Can you work these out from the model? Positions are in its coordinate system, mm. A direction names the side the tool comes from. Give positions to 0.01 mm unless a question says otherwise; leave off trailing zeros. Loops run counter-clockwise (first coordinate to the right, second up) from the corner with the lowest first, then second, coordinate; pieces in that order, holes last. Notation, with made-up numbers: (-14, -32) -> (18, -32) arc R20 ccw to (18, -27) -> close; hole circle Ø8 at (-1.5, 19). An arc over 180 degrees is marked (long way). Use CSV: the item, a comma, the result in double quotes.
from build123d import *

# Parameters (mm, degrees)
F0_W        = 45
F0_H        = 70
F1_DEPTH    = 3
F2_W        = 45
F2_H        = 4
F3_DEPTH    = 30
F4_T1_DEPTH = 119
F5_W        = 45
F5_H        = 3
F6_DEPTH    = 20
F7_R        = 5


# Not quite as in the source:
# - a fillet or chamfer that OpenCascade refuses, or shapes differently, is made with other operations: its cross-section is extruded or revolved along the edge and cut away or added


with BuildPart() as f1:
    # F0 (on Top) → F1 (new body)
    with BuildSketch(Plane.XY):
        Rectangle(F0_W, F0_H)
    extrude(amount=F1_DEPTH)

    # F2 (on face) → F3 (join)
    with BuildSketch(Plane.XY.offset(3)):
        with Locations((0, 33)):
            Rectangle(F2_W, F2_H)
    extrude(amount=F3_DEPTH)

    # F4: fillet of radius 23 on 2 edges, made by hand

    # F4_s2 → F4_t1 (cut)
    with BuildSketch(Plane.XZ.offset(-92.5)):
        with BuildLine():
            ThreePointArc((-22.5, 10), (-15.7634559673, 26.2634559673), (0.5, 33))
            Line((0.5, 33), (-22.5, 33))
            Line((-22.5, 33), (-22.5, 10))
        make_face()
        with BuildLine():
            ThreePointArc((-0.5, 33), (15.7634559673, 26.2634559673), (22.5, 10))
            Line((22.5, 10), (22.5, 33))
            Line((22.5, 33), (-0.5, 33))
        make_face()
    extrude(amount=F4_T1_DEPTH, mode=Mode.SUBTRACT)

    # F5 (on face) → F6 (join)
    with BuildSketch(Plane.XY.offset(3)):
        with Locations((0, -33.5)):
            Rectangle(F5_W, F5_H)
    extrude(amount=F6_DEPTH)

    # F7
    f7_edges = [f1.edges().sort_by_distance(p)[0] for p in [
        (-22.5, -33.5, 23),
        (22.5, -33.5, 23),
    ]]
    fillet(f7_edges, radius=F7_R)


solid = f1.part
(1) If we section it at D-D, the plane z = 14: Write out the boundary of the cut face in (x, y), then the cut area to 3 significant figures.
Answer sheet:
outline,"(-22.5, -35) -> (22.5, -35) -> (22.5, -32) -> (-22.5, -32) -> close; (-22.15, 31) -> (22.15, 31) -> (22.15, 35) -> (-22.15, 35) -> close"
area,"312 mm2"
(2) Will these pins go through, and if not, where does the flat tip stop? pin 1 Ø2 at (y, z) = (-4, 5) entering from -X; pin 2 Ø8 at (x, y) = (8.5, 11) entering from +Z; pin 3 Ø1.5 at (x, y) = (-8, -33.5) entering from +Z.
Answer sheet:
pin 1,"passes through"
pin 2,"stops at z = 3"
pin 3,"stops at z = 23"
(3) Which directions (+Z, -Z, +X, -X, +Y, -Y) give clear straight access to the entire face, cutting with the end or side of a thin tool? Please do faces 5 (the face through (0, -33, 23)), 6 (the face through (0, 0, 0)), 7 (the face through (0, 31, 14)), 8 (the face through (-16.11, 33.03, 25.91)), 9 (the face through (15.764, 33.028, 26.263)).
Answer sheet:
face 5,"+Z, +X, -X, -Y"
face 6,"-Z, +X, -X, +Y, -Y"
face 7,"+Z, +X, -X"
face 8,"+Z, -X, +Y"
face 9,"+Z, +X, +Y"
(4) If we section it at B-B, the plane x = -4.5: Write out the boundary of the cut face in (y, z).
Answer sheet:
outline,"(-35, 0) -> (35, 0) -> (35, 32.45) -> (31, 32.45) -> (31, 3) -> (-32, 3) -> (-32, 23) -> (-35, 23) -> close"
(5) If I drill on L1, parallel to Y at x = -7, z = 15; L2, parallel to Z at x = 8, y = -24; L3, parallel to Y at x = -5.5, z = 25.5, over which ranges is the centre line in solid material (lowest first)? Write a range as from..to.
Answer sheet:
L1,"y = -35..-32, 31..35"
L2,"z = 0..3"
L3,"y = 31..35"
(6) If we section it at C-C, the plane y = 5.5: Write out the boundary of the cut face in (x, z), then the cut area to 3 significant figures.
Answer sheet:
outline,"(-22.5, 0) -> (22.5, 0) -> (22.5, 3) -> (-22.5, 3) -> close"
area,"135 mm2"
(7) If we section it at A-A, the plane z = 9: Write out the boundary of the cut face in (x, y), then the cut area to 3 significant figures.
Answer sheet:
outline,"(-22.5, -35) -> (22.5, -35) -> (22.5, -32) -> (-22.5, -32) -> close; (-22.5, 31) -> (22.5, 31) -> (22.5, 35) -> (-22.5, 35) -> close"
area,"315 mm2"
(8) We'd pull the mould along Y, two halves only. Please class faces 1 (the face through (0, 0, 3)), 2 (the face through (-21.07, -33.48, 21.5)), 3 (the face through (0, 35, 13)), 4 (the face through (0, -32, 13)): released by +Y, released by -Y, zero draft, split by the parting line, or undercut.
Answer sheet:
face 1,"undercut"
face 2,"zero draft"
face 3,"released by +Y"
face 4,"undercut"
